Read the model definition and answer for the solid it produces. Units are mm, in the model's axes. Face numbers are marked on the shaded views. A direction names the side the tool comes from. Coordinates: 2 decimals unless noted, no trailing zeros. Write each loop counter-clockwise with the first axis right and the second up, starting at its lowest first coordinate (ties: lowest second). Pieces come first, ordered by that corner, then holes. Notation, with made-up numbers: (59, 75) -> (118, 75) arc R30 cw to (118, 105) -> close; hole circle Ø3 at (63, 0). An arc over 180 degrees is marked (long way). Answer in a Markdown table with one row per item. Add a question column.
Item 1: Section A-A on x = -27.5 is taken. Write down the section's boundary in (y, z), then the cut area to 3 significant figures.
Item 2: Given pin 1 Ø10 at (x, z) = (14.5, 12) entering from -Y; pin 2 Ø3 at (y, z) = (0, 16.5) entering from -X; pin 3 Ø1.6 at (x, z) = (39.5, 10) entering from +Y, each flat-ended and moving along its own axis, determine where each tip first touches the part or whether it passes through.
Item 3: Section C-C on z = 7.25 is taken. Write down the section's boundary in (x, y).
Item 4: Straight lines are drawn through the part: line 1 (Y direction, x = -4.5, z = 4.75); line 2 (X direction, y = 4, z = 14.5); line 3 (Y direction, x = 31, z = 13.5). For each, find the intervals that lie inside material, in ascending order. Write a range as from..to.
Item 5: Section B-B on y = 4 is taken. Write down the section's boundary in (x, z).
Item 6: Which of the six approach directions +Z, -Z, +X, -X, +Y, -Y give full straight-line access (tool end or side, diameter ignored) to the marked faces 5, 6, 7, 8 and 9?
Item 7: For a pull along Y with two mould halves and no side action, classify the marked faces 1, 2, 3 and 4 as +Y half, -Y half, draft (parallel to the pull), parting line (faces both ways), or undercut.
Item 8: Section D-D on y = -7 is taken. Write down the section's boundary in (x, z), then the cut area to 3 significant figures.
```python
from build123d import *

# Parameters (mm, degrees)
F0_W         = 35
F0_H         = 2
F0_W_2       = 2
F0_H_2       = 4
F1_DEPTH     = 20
F2_R         = 4.99999
F3_R         = 5
F4_R         = 2
F5_T1_DEPTH  = 43.9093010689
F5_S5_W      = 2
F5_S5_H      = 2
F5_T6_DEPTH  = 2
F5_S11_W     = 2
F5_S11_H     = 2
F5_T12_DEPTH = 2


# Not quite as in the source:
# - a fillet or chamfer that OpenCascade refuses, or shapes differently, is made with other operations: its cross-section is extruded or revolved along the edge and cut away or added
# - a fillet or chamfer is up to 0.001 mm smaller than in the source, because OpenCascade refuses the exact size


with BuildPart() as f1:
    # F0 (on Top) → F1 (new body)
    with BuildSketch(Plane.XY):
        with Locations((-20.4546505344, 18.25)):
            Rectangle(F0_W, F0_H)
        Polygon((2.9546505344, 2.5), (2.9546505344, 19.25), (-2.9546505344, 19.25), (-2.9546505344, 17.25), (-2.9546505344, -17.25), (-2.9546505344, -19.25), (2.9546505344, -19.25), (2.9546505344, -2.5), align=None)
        Polygon((38.9546505344, 2.5), (2.9546505344, 2.5), (2.9546505344, -2.5), (40.9546505344, -2.5), (40.9546505344, 2.5), align=None)
        with Locations((39.9546505344, 4.5)):
            Rectangle(F0_W_2, F0_H_2)
        with Locations((-20.4546505344, -18.25)):
            Rectangle(F0_W, F0_H)
    extrude(amount=F1_DEPTH)

    # F2 (radius 5 in the source; OpenCascade refuses exactly that, so slightly less here)
    f2_edges = [f1.edges().sort_by_distance(p)[0] for p in [
        (20.954651, 2.5, 20),
        (20.954651, 2.5, 0),
    ]]
    fillet(f2_edges, radius=F2_R)

    # F3
    f3_edges = [f1.edges().sort_by_distance(p)[0] for p in [
        (39.954651, 6.5, 20),
        (39.954651, 6.5, 0),
    ]]
    fillet(f3_edges, radius=F3_R)

    # F4
    f4_edges = [f1.edges().sort_by_distance(p)[0] for p in [
        (2.954651, 10.875, 20),
        (2.954651, -10.875, 20),
        (2.954651, 10.875, 0),
        (2.954651, -10.875, 0),
        (2.954651, 19.25, 10),
        (2.954651, -19.25, 10),
    ]]
    fillet(f4_edges, radius=F4_R)

    # F5: fillet of radius 2 on 2 edges, made by hand

    # F5_s2 → F5_t1 (cut)
    with BuildSketch(Plane.YZ.offset(-42.9546505344)):
        with BuildLine():
            ThreePointArc((17.25, 0), (18.6642135624, 0.5857864376), (19.25, 2))
            Line((19.25, 2), (19.25, 0))
            Line((19.25, 0), (17.25, 0))
        make_face()
        with BuildLine():
            ThreePointArc((19.25, 18), (18.6642135624, 19.4142135624), (17.25, 20))
            Line((17.25, 20), (19.25, 20))
            Line((19.25, 20), (19.25, 18))
        make_face()
    extrude(amount=F5_T1_DEPTH, mode=Mode.SUBTRACT)


with BuildPart() as f5_tool4:
    # F5_s5 → F5_t6 (new body)
    with BuildSketch(Plane.XZ.offset(-17.25)):
        with Locations((1.9546505344, 19)):
            Rectangle(F5_S5_W, F5_S5_H)
    extrude(amount=-F5_T6_DEPTH)

    # F5_s7 → F5_t8 (revolve, cut)
    with BuildSketch(Plane(origin=(0.9546505344, 17.25, 18), x_dir=(-0.7071067812, 0, -0.7071067812), z_dir=(0.7071067812, 0, -0.7071067812))):
        with BuildLine():
            ThreePointArc((0, -2), (2, 0), (0, 2))
            Line((0, 2), (0, -2))
        make_face()
    revolve(axis=Axis((0.9546505344, 17.25, 18), (0, 1, 0)), mode=Mode.SUBTRACT)


with BuildPart() as f1_1:
    add(f1.part)

    # F5_t3: cut F5_tool4
    add(f5_tool4.part, mode=Mode.SUBTRACT)


with BuildPart() as f5_tool10:
    # F5_s11 → F5_t12 (new body)
    with BuildSketch(Plane.XY.offset(2)):
        with Locations((1.9546505344, 18.25)):
            Rectangle(F5_S11_W, F5_S11_H)
    extrude(amount=-F5_T12_DEPTH)

    # F5_s13 → F5_t14 (revolve, cut)
    with BuildSketch(Plane(origin=(0.9546505344, 17.25, 2), x_dir=(-0.7071067812, -0.7071067812, 0), z_dir=(0.7071067812, -0.7071067812, 0))):
        with BuildLine():
            ThreePointArc((0, -2), (2, 0), (0, 2))
            Line((0, 2), (0, -2))
        make_face()
    revolve(axis=Axis((0.9546505344, 17.25, 2), (0, 0, -1)), mode=Mode.SUBTRACT)


with BuildPart() as f1_2:
    add(f1_1.part)

    # F5_t9: cut F5_tool10
    add(f5_tool10.part, mode=Mode.SUBTRACT)


solid = f1_2.part
```
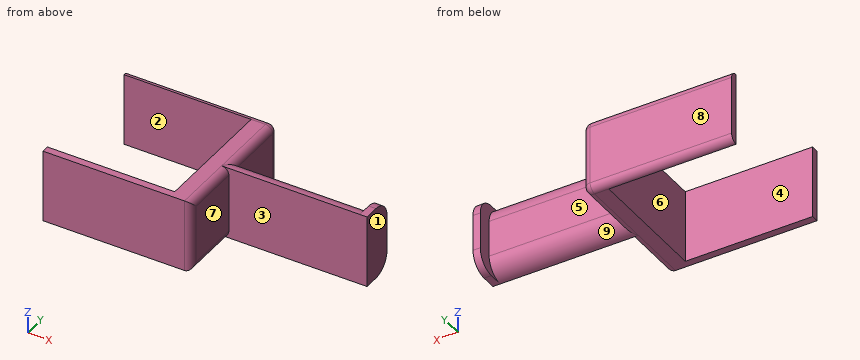
Results below:
| question | item | result |
|---|---|---|
| 1 | outline | (-19.25, 0) -> (-17.25, 0) -> (-17.25, 20) -> (-19.25, 20) -> close; (17.25, 0) arc R2 ccw to (19.25, 2) -> (19.25, 18) arc R2 ccw to (17.25, 20) -> close |
| 1 | area | 78.3 mm2 |
| 2 | pin 1 | stops at y = -2.5 |
| 2 | pin 2 | stops at x = -2.95 |
| 2 | pin 3 | stops at y = 6.5 |
| 3 | outline | (-37.95, -19.25) -> (0.95, -19.25) arc R2 ccw to (2.95, -17.25) -> (2.95, -2.5) -> (40.95, -2.5) -> (40.95, 6.5) -> (38.95, 6.5) -> (38.95, 2.5) -> (2.95, 2.5) -> (2.95, 17.25) arc R2 ccw to (0.95, 19.25) -> (-37.95, 19.25) -> (-37.95, 17.25) -> (-2.95, 17.25) -> (-2.95, -17.25) -> (-37.95, -17.25) -> close |
| 4 | line 1 | y = -19.25..-17.25, 17.25..19.25 |
| 4 | line 2 | x = -2.95..2.95, 38.95..40.95 |
| 4 | line 3 | y = -2.5..2.5 |
| 5 | outline | (-2.95, 0) -> (0.95, 0) arc R2 ccw to (2.95, 2) -> (2.95, 18) arc R2 ccw to (0.95, 20) -> (-2.95, 20) -> close; (38.95, 0.67) -> (40.95, 0.67) -> (40.95, 19.33) -> (38.95, 19.33) -> close |
| 6 | face 5 | +Z, -Z, +Y |
| 6 | face 6 | +Z, -Z, -X |
| 6 | face 7 | +Z, -Z, +X, -Y |
| 6 | face 8 | +Z, -Z, +X, -X, +Y |
| 6 | face 9 | -Z, +Y |
| 7 | face 1 | draft |
| 7 | face 2 | undercut |
| 7 | face 3 | -Y half |
| 7 | face 4 | undercut |
| 8 | outline | (-2.95, 0) -> (0.95, 0) arc R2 ccw to (2.95, 2) -> (2.95, 18) arc R2 ccw to (0.95, 20) -> (-2.95, 20) -> close |
| 8 | area | 116 mm2 |
